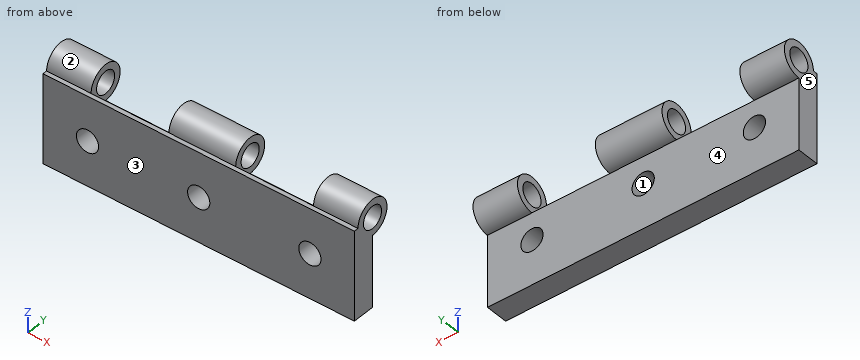
```python
from build123d import *

# Parameters (mm, degrees)
SKETCH2_W           = 88.9
SKETCH2_H           = 25.4
SKETCH2_R           = 3.175
BOSS_EXTRUDE1_DEPTH = 6.35
SKETCH3_R           = 5.08
CUT_EXTRUDE1_DEPTH  = 93.675198948
SKETCH4_R           = 5.08
SKETCH4_R_2         = 3.175
BOSS_EXTRUDE2_DEPTH = 12.7
SKETCH5_R           = 5.08
SKETCH5_R_2         = 3.175
BOSS_EXTRUDE3_DEPTH = 9.525


with BuildPart() as part:
    # Sketch2 → Boss-Extrude1 (new body)
    with BuildSketch(Plane(origin=(0, 0, 0), x_dir=(1, 0, 0), z_dir=(0, 1, 0))):
        with Locations((0, 12.7)):
            Rectangle(SKETCH2_W, SKETCH2_H)
        with Locations(Location((-31.75, 12.7, 0), (0, 0, 270))):
            Circle(SKETCH2_R, mode=Mode.SUBTRACT)
        with Locations(Location((0, 12.7, 0), (0, 0, 270))):
            Circle(SKETCH2_R, mode=Mode.SUBTRACT)
        with Locations(Location((31.75, 12.7, 0), (0, 0, 270))):
            Circle(SKETCH2_R, mode=Mode.SUBTRACT)
    extrude(amount=BOSS_EXTRUDE1_DEPTH)

    # Sketch3 → Cut-Extrude1 (cut, through all)
    with BuildSketch(Plane.ZY.offset(44.45)):
        with Locations((0, 6.35)):
            Circle(SKETCH3_R)
    extrude(amount=-CUT_EXTRUDE1_DEPTH, mode=Mode.SUBTRACT)

    # Sketch4 → Boss-Extrude2 (add)
    with BuildSketch(Plane.ZY.offset(44.45)):
        with Locations((0, 6.35)):
            Circle(SKETCH4_R)
        with Locations((0, 6.35)):
            Circle(SKETCH4_R_2, mode=Mode.SUBTRACT)
    boss_extrude2 = extrude(amount=-BOSS_EXTRUDE2_DEPTH)

    # Mirror1: Boss-Extrude2 across plane
    add(boss_extrude2.mirror(Plane(origin=(0, 0, 0), x_dir=(0, 0, 1), z_dir=(1, 0, 0))))

    # Sketch5 → Boss-Extrude3 (add, symmetric)
    with BuildSketch(Plane(origin=(0, 0, 0), x_dir=(0, 0, -1), z_dir=(1, 0, 0))):
        with Locations((0, 6.35)):
            Circle(SKETCH5_R)
        with Locations(Location((0, 6.35, 0), (0, 0, 180))):
            Circle(SKETCH5_R_2, mode=Mode.SUBTRACT)
    extrude(amount=BOSS_EXTRUDE3_DEPTH, both=True)


solid = part.part
```
Geometry check sheet. Reference: the model listing, model coordinates, mm. Face numbers are marked on the shaded views. A direction names the side the tool comes from. Coordinates: 2 decimals unless noted, no trailing zeros. Write each loop counter-clockwise with the first axis right and the second up, starting at its lowest first coordinate (ties: lowest second). Pieces come first, ordered by that corner, then holes. Notation, with made-up numbers: M -9.75,-16 L 39.25,-16 A18 ccw 39.25,15 Z; hole C 35.25,71.25 d9. An arc over 180 degrees is marked long. One line per item, written item: value. Start each with the question number.
(1) Sectioned sample at B-B, the plane z = -12.7. Enter the section's corners in (x, y) (3 decimals).
(2) Release check for a two-part mould opening along Z. For the marked faces 1, 2 and 3 record: released by +Z, released by -Z, zero draft, split by the parting line, or undercut.
(3) Tool access check on the marked faces 4 and 5. Record the directions out of +Z, -Z, +X, -X, +Y, -Y that give a thin tool (end or side, any length) a straight path to the whole face; none if there is none.
(4) Sectioned sample at C-C, the plane y = 5. Enter the section's corners in (x, z) (3 decimals), and give its area (3 significant figures).
(5) Depth check by flat-ended pin: pin 1 (5.5 mm diameter, centred on x = -31.75, z = -12.7, fed in from -Y); pin 2 (10 mm diameter, centred on x = 31.75, z = -12.7, fed in from +Y); pin 3 (8.5 mm diameter, centred on x = 0, z = -12.7, fed in from +Y). Enter the tip coordinate at first touch or a pass-through.
(6) Scan lines: line 1 along X through (y, z) = (1.75, -1.5) (3 decimals); line 2 along X through (y, z) = (2, -12.7) (3 decimals); line 3 along Y through (x, z) = (33.5, -22.5). Record each from-to range of solid material in increasing order. Write a range as [from, to].
(7) Sectioned sample at A-A, the plane x = 0. Enter the section's corners in (y, z) (3 decimals).
(8) Sectioned sample at D-D, the plane x = -13.5. Enter the section's corners in (y, z), and give its area (3 significant figures).
Filled sheet:
1. outline: M -44.45,0 L -34.925,0 L -34.925,6.35 L -44.45,6.35 Z; M -28.575,0 L -3.175,0 L -3.175,6.35 L -28.575,6.35 Z; M 3.175,0 L 28.575,0 L 28.575,6.35 L 3.175,6.35 Z; M 34.925,0 L 44.45,0 L 44.45,6.35 L 34.925,6.35 Z
2. face 1: undercut
2. face 2: split by the parting line
2. face 3: zero draft
3. face 4: -Z, +X, -X, +Y
3. face 5: +Z, -Z, -X, +Y, -Y
4. outline: M -44.45,-25.4 L 44.45,-25.4 L 44.45,-2.874 L 31.75,-2.874 L 31.75,-4.897 L 9.525,-4.897 L 9.525,-2.874 L -9.525,-2.874 L -9.525,-4.897 L -31.75,-4.897 L -31.75,-2.874 L -44.45,-2.874 Z; M -44.45,2.874 L -31.75,2.874 L -31.75,4.897 L -44.45,4.897 Z; M -9.525,2.874 L 9.525,2.874 L 9.525,4.897 L -9.525,4.897 Z; M 31.75,2.874 L 44.45,2.874 L 44.45,4.897 L 31.75,4.897 Z; hole C -31.75,-12.7 d6.35; hole C 0,-12.7 d6.35; hole C 31.75,-12.7 d6.35
4. area: 1,910 mm²
5. pin 1: through
5. pin 2: y = 6.35
5. pin 3: y = 6.35
6. line 1: [-44.45, -31.75], [-9.525, 9.525], [31.75, 44.45]
6. line 2: [-44.45, -34.925], [-28.575, -3.175], [3.175, 28.575], [34.925, 44.45]
6. line 3: [0, 6.35]
7. outline: M 0,-25.4 L 6.35,-25.4 L 6.35,-15.875 L 0,-15.875 Z; M 0,-9.525 L 6.35,-9.525 L 6.35,-5.08 A5.08 ccw long 1.27,0 L 0,0 Z; hole C 6.35,0 d6.35
8. outline: M 0,-25.4 L 6.35,-25.4 L 6.35,-5.08 A5.08 cw 1.27,0 L 0,0 Z
8. area: 141 mm²
